```python
from build123d import *

# Parameters (mm, degrees)
SKETCH1_W           = 21.43125
SKETCH1_H           = 107.553125
SKETCH1_R           = 4.7625
SKETCH1_R_2         = 2.38125
BOSS_EXTRUDE3_DEPTH = 15.875
FILLET1_R           = 3.175
FILLET2_R           = 3.175
FILLET3_R           = 3.175
FILLET4_R           = 3.175
SKETCH3_W           = 9.525
SKETCH3_H           = 76.2
CUT_EXTRUDE2_DEPTH  = 111.810598766
FILLET5_R           = 4.7625
FILLET6_R           = 4.7625
SKETCH5_R           = 2.38125
CUT_EXTRUDE3_DEPTH  = 21.43125


with BuildPart() as part:
    # Sketch1 → Boss-Extrude3 (new body)
    with BuildSketch(Plane.XY):
        with Locations((10.715625, 53.7765625)):
            Rectangle(SKETCH1_W, SKETCH1_H)
        with Locations((10.484595663, 10.31875)):
            Circle(SKETCH1_R, mode=Mode.SUBTRACT)
        with Locations((10.484595663, 99.21875)):
            Circle(SKETCH1_R_2, mode=Mode.SUBTRACT)
        with Locations((10.484595663, 86.51875)):
            Circle(SKETCH1_R_2, mode=Mode.SUBTRACT)
        with Locations((10.484595663, 73.81875)):
            Circle(SKETCH1_R_2, mode=Mode.SUBTRACT)
        with Locations((10.484595663, 61.11875)):
            Circle(SKETCH1_R_2, mode=Mode.SUBTRACT)
        with Locations((10.484595663, 48.41875)):
            Circle(SKETCH1_R_2, mode=Mode.SUBTRACT)
    extrude(amount=BOSS_EXTRUDE3_DEPTH)

    # Fillet1
    fillet1_edges = [part.edges().sort_by_distance(p)[0] for p in [
        (21.43125, 0, 7.9375),
    ]]
    fillet(fillet1_edges, radius=FILLET1_R)

    # Fillet2
    fillet2_edges = [part.edges().sort_by_distance(p)[0] for p in [
        (0, 0, 7.9375),
    ]]
    fillet(fillet2_edges, radius=FILLET2_R)

    # Fillet3
    fillet3_edges = [part.edges().sort_by_distance(p)[0] for p in [
        (21.43125, 107.553125, 7.9375),
    ]]
    fillet(fillet3_edges, radius=FILLET3_R)

    # Fillet4
    fillet4_edges = [part.edges().sort_by_distance(p)[0] for p in [
        (0, 107.553125, 7.9375),
    ]]
    fillet(fillet4_edges, radius=FILLET4_R)

    # Sketch3 → Cut-Extrude2 (cut, through all)
    with BuildSketch(Plane(origin=(0, 0, 0), x_dir=(0, 0, -1), z_dir=(1, 0, 0))):
        with Locations((-7.9375, 69.453125)):
            Rectangle(SKETCH3_W, SKETCH3_H)
    extrude(amount=CUT_EXTRUDE2_DEPTH, mode=Mode.SUBTRACT)

    # Fillet5
    fillet5_edges = [part.edges().sort_by_distance(p)[0] for p in [
        (10.715625, 31.353125, 3.175),
    ]]
    fillet(fillet5_edges, radius=FILLET5_R)

    # Fillet6
    fillet6_edges = [part.edges().sort_by_distance(p)[0] for p in [
        (10.715625, 31.353125, 12.7),
    ]]
    fillet(fillet6_edges, radius=FILLET6_R - 0.0001)  # a hair under: the kernel refuses the full size

    # Sketch5 → Cut-Extrude3 (cut)
    with BuildSketch(Plane(origin=(0, 0, 0), x_dir=(0, 0, -1), z_dir=(1, 0, 0))):
        with Locations(Location((-7.9375, 10.20445, 0), (0, 0, 180))):
            Circle(SKETCH5_R)
    extrude(amount=CUT_EXTRUDE3_DEPTH, mode=Mode.SUBTRACT)


solid = part.part
```
Verification items for the finished model (mm, model axes). A direction names the side the tool comes from. Give positions to 0.01 mm unless a question says otherwise; leave off trailing zeros. Loops run counter-clockwise (first coordinate to the right, second up) from the corner with the lowest first, then second, coordinate; pieces in that order, holes last. Notation, with made-up numbers: M 46.5,44.5 L 84.5,44.5 A25 cw 84.5,81.5 Z; hole C 41,-7 d4. An arc over 180 degrees is marked long. Return JSON: item names as keys, results as strings.
1) Tool access check on faces 3 (the flat face through (11, 71, 3.175)), 4 (the cylindrical face through (10.17, 63.48, 14.27)). Record the directions out of +Z, -Z, +X, -X, +Y, -Y that give a thin tool (end or side, any length) a straight path to the whole face; none if there is none.
Findings:
{"face 3": "+X, -X, +Y", "face 4": "+Z, -Z"}
2) Section check D-D, the plane z = 14.75. Count the separate pieces of the cut face and the enclosed holes in it, and give its area (3 significant figures).
Findings:
{"separate pieces": "1", "enclosed holes": "6", "area": "2,140 mm2"}
3) Mould release check, pull along Z, two halves, no side actions. Record for faces 1 (the flat face through (11, 71, 12.7)), 2 (the cylindrical face through (0.955, 106.648, 14.31)): released by +Z, released by -Z, zero draft, split by the parting line, or undercut.
Findings:
{"face 1": "undercut", "face 2": "zero draft"}
4) Material ranges on L1, parallel to Z at x = 3, y = 83.5 (3 decimals); L2, parallel to Y at x = 11.25, z = 5.5; L3, parallel to Y at x = 7.75, z = 4.25, recorded low to high. Write a range as [from, to].
Findings:
{"L1": "z = [0, 3.175], [12.7, 15.875]", "L2": "y = [0, 5.62], [15.02, 32.02]", "L3": "y = [0, 6.42], [14.22, 33.1]"}
5) Section check A-A, the plane y = 69. Enter the section's corners in (x, z) (3 decimals), and give its area (3 significant figures).
Findings:
{"outline": "M 0,0 L 21.431,0 L 21.431,3.175 L 0,3.175 Z; M 0,12.7 L 21.431,12.7 L 21.431,15.875 L 0,15.875 Z", "area": "136 mm2"}
6) Gauge pin test, flat ends, axial feed: P1, Ø5.5, axis at x = 10.48, y = 10.32, coming from the +Z side; P2, Ø1, axis at x = 18, z = 3.5, coming from the +Y side. Record the tip position at first contact, or that the pin passes through.
Findings:
{"P1": "passes through", "P2": "stops at y = 107.55"}
